Autodesk Fusion 360 part; units mm, degrees
sketch "Esquisse1" plane through (0, 0, 0) normal (0, 0, 1) x (1, 0, 0)
  line L0 (60, -86) -> (-60, -86)
  line L1 (-60, -86) -> (-60, 86)
  line L2 (-60, 86) -> (60, 86)
  line L3 (60, 86) -> (60, -86)
  line L4 (60, -86) -> (-60, 86) construction
  line L5 (-60, -86) -> (60, 86) construction
  dimension "d1" = 120
  dimension "d2" = 172
sketch "Esquisse2" plane through (0, 0, 0) normal (0, 0, 1) x (1, 0, 0)
  line L0 (0, -86) -> (0, -101)
  line L1 (0, 86) -> (0, 101)
  line L2 (60, -86) -> (-60, -86)
  line L3 (-60, -86) -> (-60, -116)
  line L4 (-60, -116) -> (60, -116)
  line L5 (60, -116) -> (60, -86)
  line L6 (60, -86) -> (-60, -116) construction
  line L7 (-60, -86) -> (60, -116) construction
  line L8 (-60, 86) -> (60, 86)
  line L9 (60, 86) -> (60, 116)
  line L10 (60, 116) -> (-60, 116)
  line L11 (-60, 116) -> (-60, 86)
  line L12 (-60, 86) -> (60, 116) construction
  line L13 (60, 86) -> (-60, 116) construction
  arc A0 (60, 86) -> (-60, 86) centre (0, -26.5) ccw
  arc A1 (-60, -86) -> (60, -86) centre (0, 26.5) ccw
  point P0 (0, -101)
  point P1 (0, 101)
  dimension "d3" = 15
  dimension "d4" = 15
extrude "Extrusion1" add sketch "Esquisse1" sketch "Esquisse2" along normal blind 10 of sketch 2 contours L0 L2 A1 | L0 L2 A1 | L1 L8 A0 | L1 L8 A0
sketch "Esquisse3" plane through (0, 0, 10) normal (0, 0, 1) x (-1, 0, 0)
  line L0 (60, -86) -> (60, 86)
  arc A0 (60, 86) -> (-60, 86) centre (0, -26.5) ccw
  line L1 (-60, 86) -> (-60, -86)
  arc A1 (-60, -86) -> (60, -86) centre (0, 26.5) ccw
  line L2 (60, 86) -> (-60, 86)
  line L3 (60, -86) -> (-60, -86)
  line L4 (-60, 86) -> (-60, 70)
  line L5 (-60, 70) -> (-60, 48)
  line L6 (-60, 48) -> (-60, -48)
  line L7 (-60, -48) -> (-60, -70)
  line L8 (60, 86) -> (60, 70)
  line L9 (60, 70) -> (60, 48)
  line L10 (60, 48) -> (60, -48)
  line L11 (60, -48) -> (60, -70)
  line L12 (60, 70) -> (36, 70)
  line L13 (36, 70) -> (36, 48)
  line L14 (36, 48) -> (60, 48)
  line L15 (60, -70) -> (36, -70)
  line L16 (36, -70) -> (36, -48)
  line L17 (36, -48) -> (60, -48)
  line L18 (-60, -70) -> (-36, -70)
  line L19 (-36, -70) -> (-36, -48)
  line L20 (-36, -48) -> (-60, -48)
  line L21 (-60, 70) -> (-36, 70)
  line L22 (-36, 70) -> (-36, 48)
  line L23 (-60, 48) -> (-36, 48)
  dimension "d7" = 16
  dimension "d8" = 22
  dimension "d9" = 96
  dimension "d10" = 22
  dimension "d11" = 16
  dimension "d12" = 22
  dimension "d13" = 96
  dimension "d14" = 22
  dimension "d15" = 24
  dimension "d16" = 24
  dimension "d17" = 22
sketch "Esquisse4" plane through (0, 0, 10) normal (0, 0, 1) x (-1, 0, 0)
  line L0 (-60, -86) -> (-17, -86)
  line L1 (-17, -86) -> (17, -86)
  line L2 (17, -86) -> (17, -70)
  line L3 (17, -70) -> (-17, -70)
  line L4 (-17, -70) -> (-17, -86)
  dimension "d18" = 43
  dimension "d19" = 34
extrude "Extrusion2" cut sketch "Esquisse3" against normal blind 5
extrude "Extrusion3" cut sketch "Esquisse4" along normal blind 0 and the other way blind 25
sketch "Esquisse5" plane through (0, 0, 5) normal (0, 0, 1) x (-1, 0, 0)
  arc A0 (60, 86) -> (-60, 86) centre (0, -26.5) ccw
  line L0 (-60, 86) -> (-60, -86)
  arc A1 (-60, -86) -> (60, -86) centre (0, 26.5) ccw
  line L1 (60, -86) -> (60, 86)
  line L2 (-60, 86) -> (60, 86)
  line L3 (-60, -86) -> (-60, -70)
  line L4 (-60, -70) -> (-60, -48)
  line L5 (-60, -48) -> (-60, 48)
  line L6 (-60, 48) -> (-60, 70)
  line L7 (-60, -70) -> (-36, -70)
  line L8 (-36, -70) -> (-36, -48)
  line L9 (-36, -48) -> (-60, -48)
  line L10 (-60, 70) -> (-36, 70)
  line L11 (-60, 48) -> (-36, 48)
  line L12 (-36, 48) -> (-36, 70)
  line L13 (60, -70) -> (36, -70)
  line L14 (36, -70) -> (36, -48)
  line L15 (36, -48) -> (60, -48)
  line L16 (60, 48) -> (36, 48)
  line L17 (36, 48) -> (36, 70)
  line L18 (36, 70) -> (60, 70)
  dimension "d27" = 16
  dimension "d28" = 22
  dimension "d29" = 96
  dimension "d30" = 22
  dimension "d31" = 24
  dimension "d32" = 24
sketch "Esquisse6" plane through (0, 0, 5) normal (0, 0, 1) x (-1, 0, 0)
  line L0 (27.5, -60) -> (-27.5, -60)
  line L1 (-27.5, -60) -> (-27.5, 7)
  line L2 (-27.5, 7) -> (27.5, 7)
  line L3 (27.5, 7) -> (27.5, -60)
  dimension "d34" = 55
  dimension "d35" = 67
sketch "Esquisse7" plane through (0, 0, 5) normal (0, 0, 1) x (-1, 0, 0)
  line L0 (27.5, 17) -> (-27.5, 17)
  line L1 (-27.5, 17) -> (-27.5, 83)
  line L2 (-27.5, 83) -> (27.5, 83)
  line L3 (27.5, 83) -> (27.5, 17)
  dimension "d38" = 55
  dimension "d39" = 66
sketch "Esquisse8" plane through (0, 0, 5) normal (0, 0, 1) x (-1, 0, 0)
  line L0 (17, -70) -> (-17, -70)
  line L1 (-17, -70) -> (-17, -86)
  line L2 (-17, -86) -> (17, -86)
  line L3 (17, -86) -> (17, -70)
extrude "Extrusion4" add sketch "Esquisse8" against normal blind 5
sketch "Esquisse9" plane through (0, 0, 5) normal (0, 0, 1) x (-1, 0, 0)
  line L0 (-60, -86) -> (60, -86)
Can you work these out from the model? Positions are in its coordinate system, mm. Give positions to 0.01 mm unless a question says otherwise; leave off trailing zeros. Loops run counter-clockwise (first coordinate to the right, second up) from the corner with the lowest first, then second, coordinate; pieces in that order, holes last. Notation, with made-up numbers: (-21, 71.25) - (17, 71.25) arc R23 ccw to (17, 102.25) - close; hole circle Ø9 at (25.25, -12). An arc over 180 degrees is marked (long way). Answer as a JSON object with one key per item and string values.
Q1. Imagine slicing it at B-B on x = -44. Write out the boundary of the cut face in (y, z).
Geometry says:
{"outline": "(-93.17, 0) - (93.17, 0) - (93.17, 5) - (-93.17, 5) - close"}
Q2. Imagine slicing it at A-A on z = 3.7. Write out the boundary of the cut face in (x, y).
Geometry says:
{"outline": "(-60, -86) arc R127.5 ccw to (60, -86) - (60, 86) arc R127.5 ccw to (-60, 86) - close"}
Q3. Will these pins go through, and if not, where does the flat tip stop? P1, Ø3, axis at x = -32, z = 3, coming from the +Y side; P2, Ø3, axis at x = -13, z = 3.5, coming from the -Y side; P3, Ø2, axis at x = -42, z = 1.5, coming from the +Y side.
Geometry says:
{"P1": "y = 97.3", "P2": "y = -100.48", "P3": "y = 94.23"}
Q4. If I drill on L1, parallel to Y at x = -49.5, z = 1.6; L2, parallel to Y at x = 9, z = 2.75; L3, parallel to X at y = -89, z = 0.8, over which ranges is the centre line in solid material (lowest first)?
Geometry says:
{"L1": "-91 to 91", "L2": "-100.68 to 100.68", "L3": "-54 to 54"}
